Check sheet for the modelled part. Datum: model origin and axes. Units: mm. A direction names the side the tool comes from. Give positions to 0.01 mm unless a question says otherwise; leave off trailing zeros. Write each loop counter-clockwise with the first axis right and the second up, starting at its lowest first coordinate (ties: lowest second). Pieces come first, ordered by that corner, then holes. Notation, with made-up numbers: M 83,-20.75 L 89,-20.75 A20 ccw 89,0.25 Z; hole C 48,85.5 d9. An arc over 180 degrees is marked long. Write item = value, one per line. Start each with the question number.
1) Sectioned sample at B-B, the plane z = 8. Record the cut outline in (x, y).
2) Sectioned sample at C-C, the plane y = -3.75. Record the cut outline in (x, z), then the cut area to 3 significant figures.
3) Draft check along X on faces 5 (the face through (-54.65, 2.46, 5.44)), 6 (the face through (-63.14, 2.46, 0.25)), 7 (the face through (30, -20, 13)), 8 (the face through (-48.56, 2.46, -23.45)). Enter one of: pulls with the +X half, pulls with the -X half, needs draft (parallel to the pull), parting line crosses it, or undercut.
4) Scan lines: L1, parallel to Z at x = 2, y = 1; L2, parallel to Z at x = -33, y = -1; L3, parallel to Y at x = -58, z = -1. Record each from-to range of solid material in increasing order.
5) Set-up check for faces 1 (the face through (3, 2, -27)), 2 (the face through (0, 2, -33)), 3 (the face through (-20.246, -5, 12)), 4 (the face through (0, 0, 2)): record each of +Z, -Z, +X, -X, +Y, -Y from which the full face is reachable in a straight line by a thin tool's end or side.
6) Sectioned sample at A-A, the plane x = 28.5. Record the cut outline in (y, z).
7) Gauge pin test, flat ends, axial feed: pin 1 (2.5 mm diameter, centred on x = -4, y = 2, fed in from +Z); pin 2 (6 mm diameter, centred on x = 27, y = -13.5, fed in from -Z); pin 3 (2.5 mm diameter, centred on y = 3.5, z = -16, fed in from +X). Record the tip position at first contact, or that the pin passes through.
8) Sectioned sample at D-D, the plane z = -9. Record the cut outline in (x, y), then the cut area to 3 significant figures.
from build123d import *

# Parameters (mm, degrees)
SKETCH1_R           = 3
BOSS_EXTRUDE1_DEPTH = 5
SKETCH2_W           = 20
SKETCH2_H           = 3
BOSS_EXTRUDE2_DEPTH = 20


with BuildPart() as part:
    # Sketch1 → Boss-Extrude1 (new body)
    with BuildSketch(Plane(origin=(0, 0, 0), x_dir=(1, 0, 0), z_dir=(0, 1, 0))):
        with BuildLine():
            Line((-46.754410697, 33), (48.5, 33))
            Line((48.5, 33), (60.984651798, 31.862682764))
            ThreePointArc((60.984651798, 31.862682764), (63.227835275, 27.240115524), (66.269368613, 31.381259683))
            Line((66.269368613, 31.381259683), (73.34328665, 30.736845322))
            ThreePointArc((73.34328665, 30.736845322), (78.505606793, 26.614733634), (76.749984847, 20.246127381))
            Line((76.749984847, 20.246127381), (46.754410697, -6))
            Line((46.754410697, -6), (39.754410697, -6))
            Line((39.754410697, -6), (39.754410697, -14))
            Line((39.754410697, -14), (19.754410697, -14))
            Line((19.754410697, -14), (19.754410697, -6))
            Line((19.754410697, -6), (-20.245589303, -6))
            Line((-20.245589303, -6), (-20.245589303, -14))
            Line((-20.245589303, -14), (-40.245589303, -14))
            Line((-40.245589303, -14), (-40.245589303, -6))
            Line((-40.245589303, -6), (-48.5, -6))
            Line((-48.5, -6), (-60.984651798, -4.862682764))
            ThreePointArc((-60.984651798, -4.862682764), (-63.227835275, -0.240115524), (-66.269368613, -4.381259683))
            Line((-66.269368613, -4.381259683), (-73.34328665, -3.736845322))
            ThreePointArc((-73.34328665, -3.736845322), (-78.505606793, 0.385266366), (-76.749984847, 6.753872619))
            Line((-76.749984847, 6.753872619), (-46.754410697, 33))
        make_face()
        with Locations(Location((72.798957199, 24.76158755, 0), (0, 0, 270))):
            Circle(SKETCH1_R, mode=Mode.SUBTRACT)
        with Locations(Location((-72.798957199, 2.23841245, 0), (0, 0, 270))):
            Circle(SKETCH1_R, mode=Mode.SUBTRACT)
        Polygon((-44.5, 27), (52.5, 27), (52.5, 7), (44.5, 0), (-52.5, 0), (-52.5, 20), align=None, mode=Mode.SUBTRACT)
        Polygon((58.5, 21.65), (58.5, 12.25), (68.283497031, 20.810559902), align=None, mode=Mode.SUBTRACT)
        Polygon((-58.5, 14.75), (-68.283497031, 6.189440098), (-58.5, 5.35), align=None, mode=Mode.SUBTRACT)
    extrude(amount=BOSS_EXTRUDE1_DEPTH)

    # Sketch2 → Boss-Extrude2 (add)
    with BuildSketch(Plane.XZ):
        with Locations((-30.245589303, 12.5)):
            Rectangle(SKETCH2_W, SKETCH2_H)
        with Locations((29.754410697, 12.5)):
            Rectangle(SKETCH2_W, SKETCH2_H)
    extrude(amount=BOSS_EXTRUDE2_DEPTH)


solid = part.part
Data:
q1.outline = M -40.25,0 L -20.25,0 L -20.25,5 L -40.25,5 Z; M 19.75,0 L 39.75,0 L 39.75,5 L 19.75,5 Z
q2.outline = M -40.25,11 L -20.25,11 L -20.25,14 L -40.25,14 Z; M 19.75,11 L 39.75,11 L 39.75,14 L 19.75,14 Z
q2.area = 120 mm2
q3.face_5 = pulls with the -X half
q3.face_6 = undercut
q3.face_7 = needs draft
q3.face_8 = undercut
q4.L1 = -33 to -27, 0 to 6
q4.L2 = 11 to 14
q4.L3 = 0 to 5
q5.face_1 = +Y, -Y
q5.face_2 = -Z, +X, -X, +Y, -Y
q5.face_3 = +Z, +Y, -Y
q5.face_4 = -Z, +X, -X, -Y
q6.outline = M -20,11 L 0,11 L 0,0 L 5,0 L 5,14 L -20,14 Z; M 0,-33 L 5,-33 L 5,-27 L 0,-27 Z
q7.pin_1 = 6
q7.pin_2 = 11
q7.pin_3 = 73.33
q8.outline = M -74.18,0 L -65.07,0 L -65.07,5 L -74.18,5 Z; M -58.5,0 L -52.5,0 L -52.5,5 L -58.5,5 Z; M 52.5,0 L 63.9,0 L 63.9,5 L 52.5,5 Z
q8.area = 133 mm2
